Print and shaded views of the part. All mm, measured from the part's lowest x, y and z. A direction names the side the tool comes from. Give positions to 0.01 mm unless a question says otherwise; leave off trailing zeros. Write each loop counter-clockwise with the first axis right and the second up, starting at its lowest first coordinate (ties: lowest second). Pieces come first, ordered by that corner, then holes. Notation, with made-up numbers: (-16, 55.25) -> (38, 55.25) arc R19 ccw to (38, 60.25) -> close; hole circle Ø6 at (29, -14). An arc over 180 degrees is marked (long way). Put each result on its own line as item: value.
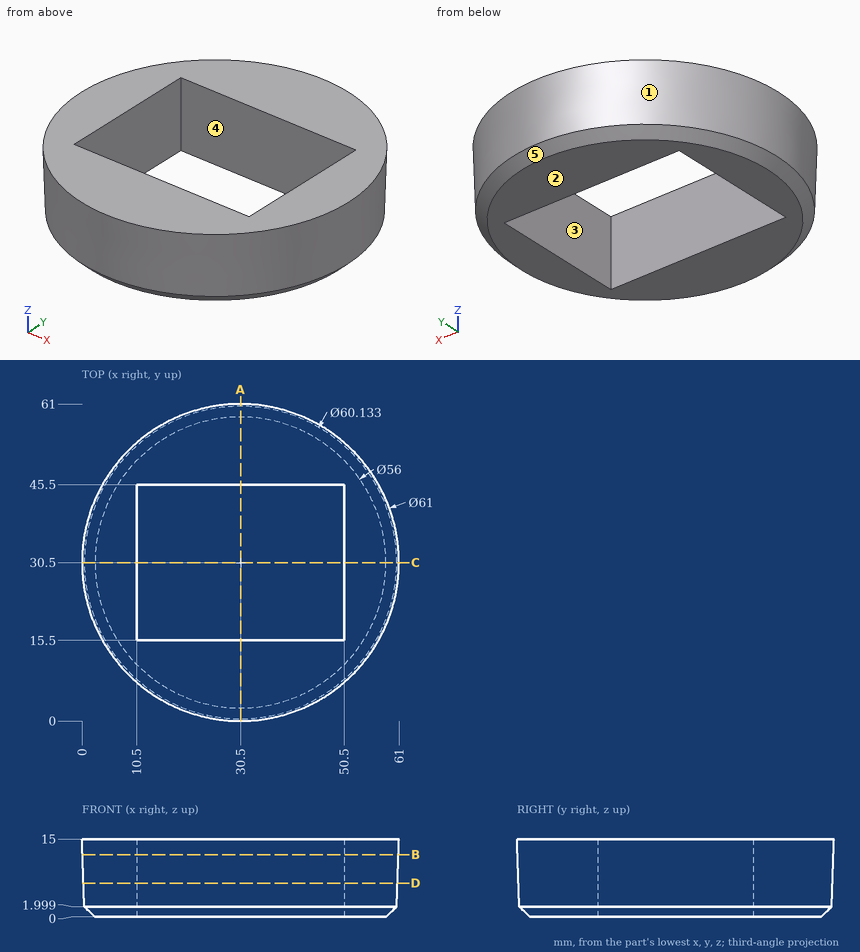
1) Tool access for the marked faces 4 and 5: list every direction of +Z, -Z, +X, -X, +Y, -Y with a clear straight run to the whole face (end or side of a thin tool).
Filled sheet:
face 4: +Z, -Z
face 5: -Z
2) Slice it at A-A (x = 30.5). Write the cut outline in (y, z).
Filled sheet:
outline: (0, 15) -> (0.43, 2) -> (2.5, 0) -> (15.5, 0) -> (15.5, 15) -> close; (45.5, 0) -> (58.5, 0) -> (60.57, 2) -> (61, 15) -> (45.5, 15) -> close
3) Wall check: L1, parallel to Y at x = 32, z = 10.25 (1 decimal); L2, parallel to Y at x = 18.5, z = 2; L3, parallel to X at y = 23, z = 5.25. Give the ranges that are in metal, low to high.
Filled sheet:
L1: 0.2 to 15.5, 45.5 to 60.8
L2: 2.93 to 15.5, 45.5 to 58.07
L3: 1.27 to 10.5, 50.5 to 59.73
4) Slice it at B-B (z = 12). Write the cut outline in (x, y).
Filled sheet:
outline: circle Ø60.8 at (30.5, 30.5); hole (10.5, 15.5) -> (50.5, 15.5) -> (50.5, 45.5) -> (10.5, 45.5) -> close
5) Pull direction X, two halves, no side cores. Call the marked faces 1, 2 and 3: released by +X, released by -X, zero draft, split by the parting line, or undercut.
Filled sheet:
face 1: split by the parting line
face 2: zero draft
face 3: undercut
6) Slice it at D-D (z = 6.5). Write the cut outline in (x, y).
Filled sheet:
outline: circle Ø60.43 at (30.5, 30.5); hole (10.5, 15.5) -> (50.5, 15.5) -> (50.5, 45.5) -> (10.5, 45.5) -> close
7) Slice it at C-C (y = 30.5). Write the cut outline in (x, z).
Filled sheet:
outline: (0, 15) -> (0.43, 2) -> (2.5, 0) -> (10.5, 0) -> (10.5, 15) -> close; (50.5, 0) -> (58.5, 0) -> (60.57, 2) -> (61, 15) -> (50.5, 15) -> close
8) Pin check, flat tips, straight feed: pin 1 (7.5 mm diameter, centred on x = 29.5, z = 5, fed in from -Y); pin 2 (1.5 mm diameter, centred on x = 14, z = 8.5, fed in from +Y); pin 3 (3 mm diameter, centred on x = 20.5, z = 4, fed in from -Y). Stop position of each tip, or through.
Filled sheet:
pin 1: y = 0.21
pin 2: y = 56.37
pin 3: y = 1.59
